The model under review builds one solid part; all positions refer to its coordinate system, in mm. A direction names the side the tool comes from. Coordinates: 2 decimals unless noted, no trailing zeros. Order: outer loops, then holes, each group sorted by start corner. A loop starts at its lowest first (then second) coordinate and runs counter-clockwise, first axis right, second up. Notation, with made-up numbers: M 23,46.25 L 73,46.25 A18 cw 73,57.25 Z; hole C -35,-26 d11. An arc over 180 degrees is marked long. Answer in a Markdown table with one row per item.
from build123d import *

# Parameters (mm, degrees)
ESQUISSE1_W             = 266.7
ESQUISSE1_H             = 38.1
BOSS_EXTRU_1_DEPTH      = 12.7
ESQUISSE2_W             = 12.7
ESQUISSE2_H             = 38.1
BOSS_EXTRU_2_DEPTH      = 279.4
ESQUISSE3_R             = 3.175
ENL_V_MAT_EXTRU_1_DEPTH = 311.176538442
ESQUISSE4_R             = 3.175
ENL_V_MAT_EXTRU_2_DEPTH = 311.176538442
BOSS_EXTRU_3_REACH      = 389.558
ESQUISSE5_W             = 38.1
ESQUISSE5_H             = 12.7
BOSS_EXTRU_4_REACH      = 389.558
ESQUISSE6_W             = 38.1
ESQUISSE6_H             = 12.7
ESQUISSE9_R             = 3.175
ENL_V_MAT_EXTRU_3_DEPTH = 396.997730423
ESQUISSE10_R            = 2
ENL_V_MAT_EXTRU_4_DEPTH = 396.997730423
ESQUISSE12_R            = 4.7625
ENL_V_MAT_EXTRU_5_DEPTH = 4.7625
ESQUISSE13_R            = 4.7625
ENL_V_MAT_EXTRU_6_DEPTH = 4.7625
ENL_V_START             = -76.2
ESQUISSE17_R            = 3.175
ENL_V_MAT_EXTRU_7_DEPTH = 76.2
ESQUISSE18_R            = 2
ENL_V_MAT_EXTRU_8_DEPTH = 25.4
ESQUISSE20_R            = 3.96875
ENL_V_MAT_EXTRU_9_DEPTH = 4.7625


with BuildPart() as part:
    # Esquisse1 → Boss.-Extru.1 (new body)
    with BuildSketch(Plane(origin=(0, 0, 0), x_dir=(1, 0, 0), z_dir=(0, 1, 0))):
        Rectangle(ESQUISSE1_W, ESQUISSE1_H)
    extrude(amount=BOSS_EXTRU_1_DEPTH)

    # Esquisse2 → Boss.-Extru.2 (add)
    with BuildSketch(Plane(origin=(0, 12.7, 0), x_dir=(1, 0, 0), z_dir=(0, 1, 0))):
        with Locations((-127, 0)):
            Rectangle(ESQUISSE2_W, ESQUISSE2_H)
        with Locations((127, 0)):
            Rectangle(ESQUISSE2_W, ESQUISSE2_H)
    extrude(amount=BOSS_EXTRU_2_DEPTH)

    # Esquisse3 → Enlèv. mat.-Extru.1 (cut, through all)
    with BuildSketch(Plane(origin=(0, 12.7, 0), x_dir=(1, 0, 0), z_dir=(0, 1, 0))):
        with Locations(Location((-22.225, 6.35, 0), (0, 0, 270))):
            Circle(ESQUISSE3_R)
    extrude(amount=-ENL_V_MAT_EXTRU_1_DEPTH, mode=Mode.SUBTRACT)

    # Esquisse4 → Enlèv. mat.-Extru.2 (cut, through all)
    with BuildSketch(Plane(origin=(0, 12.7, 0), x_dir=(1, 0, 0), z_dir=(0, 1, 0))):
        with Locations(Location((22.225, 6.35, 0), (0, 0, 270))):
            Circle(ESQUISSE4_R)
    extrude(amount=-ENL_V_MAT_EXTRU_2_DEPTH, mode=Mode.SUBTRACT)

    # Esquisse5 → Boss.-Extru.3 (add, up to next)
    with BuildSketch(Plane(origin=(-120.65, 0, 0), x_dir=(0, 0, -1), z_dir=(1, 0, 0)), mode=Mode.PRIVATE) as boss_extru_3_sk1:
        with Locations((0, 55.5625)):
            Rectangle(ESQUISSE5_W, ESQUISSE5_H)
    boss_extru_3_tool1 = extrude(boss_extru_3_sk1.sketch, amount=BOSS_EXTRU_3_REACH, mode=Mode.PRIVATE) - part.part
    add(boss_extru_3_tool1.solids().sort_by_distance((-120.65, 55.5625, 0))[0])

    # Esquisse6 → Boss.-Extru.4 (add, up to next)
    with BuildSketch(Plane(origin=(-120.65, 0, 0), x_dir=(0, 0, -1), z_dir=(1, 0, 0)), mode=Mode.PRIVATE) as boss_extru_4_sk1:
        with Locations((0, 285.75)):
            Rectangle(ESQUISSE6_W, ESQUISSE6_H)
    boss_extru_4_tool1 = extrude(boss_extru_4_sk1.sketch, amount=BOSS_EXTRU_4_REACH, mode=Mode.PRIVATE) - part.part
    add(boss_extru_4_tool1.solids().sort_by_distance((-120.65, 285.75, 0))[0])

    # Esquisse9 → Enlèv. mat.-Extru.3 (cut, through all)
    with BuildSketch(Plane.ZY.offset(133.35)):
        with Locations((0, 254)):
            Circle(ESQUISSE9_R)
    extrude(amount=-ENL_V_MAT_EXTRU_3_DEPTH, mode=Mode.SUBTRACT)

    # Esquisse10 → Enlèv. mat.-Extru.4 (cut, through all)
    with BuildSketch(Plane.ZY.offset(133.35)):
        with Locations((8, 262)):
            Circle(ESQUISSE10_R)
        with Locations((-8, 262)):
            Circle(ESQUISSE10_R)
        with Locations((-8, 246)):
            Circle(ESQUISSE10_R)
        with Locations((8, 246)):
            Circle(ESQUISSE10_R)
    extrude(amount=-ENL_V_MAT_EXTRU_4_DEPTH, mode=Mode.SUBTRACT)

    # Esquisse12 → Enlèv. mat.-Extru.5 (cut)
    with BuildSketch(Plane.ZY.offset(133.35)):
        with Locations((8, 262)):
            Circle(ESQUISSE12_R)
        with Locations((-8, 262)):
            Circle(ESQUISSE12_R)
        with Locations((-8, 246)):
            Circle(ESQUISSE12_R)
        with Locations((8, 246)):
            Circle(ESQUISSE12_R)
    extrude(amount=-ENL_V_MAT_EXTRU_5_DEPTH, mode=Mode.SUBTRACT)

    # Esquisse13 → Enlèv. mat.-Extru.6 (cut)
    with BuildSketch(Plane(origin=(120.65, 0, 0), x_dir=(0, 0, -1), z_dir=(1, 0, 0))):
        with Locations(Location((8, 262, 0), (0, 0, 180))):
            Circle(ESQUISSE13_R)
        with Locations(Location((8, 246, 0), (0, 0, 180))):
            Circle(ESQUISSE13_R)
        with Locations(Location((-8, 246, 0), (0, 0, 180))):
            Circle(ESQUISSE13_R)
        with Locations(Location((-8, 262, 0), (0, 0, 180))):
            Circle(ESQUISSE13_R)
    extrude(amount=ENL_V_MAT_EXTRU_6_DEPTH, mode=Mode.SUBTRACT)

    # Esquisse17 → Enlèv. mat.-Extru.7 (cut)
    with BuildSketch(Plane.XZ.offset(ENL_V_START)):
        with Locations(Location((22.225, -6.35, 0), (0, 0, 90))):
            Circle(ESQUISSE17_R)
        with Locations(Location((-22.225, -6.35, 0), (0, 0, 90))):
            Circle(ESQUISSE17_R)
    extrude(amount=ENL_V_MAT_EXTRU_7_DEPTH, mode=Mode.SUBTRACT)

    # Esquisse18 → Enlèv. mat.-Extru.8 (cut)
    with BuildSketch(Plane(origin=(0, 61.9125, 0), x_dir=(1, 0, 0), z_dir=(0, 1, 0))):
        with Locations(Location((14.225, -1.65, 0), (0, 0, 270))):
            Circle(ESQUISSE18_R)
        with Locations(Location((14.225, 14.35, 0), (0, 0, 270))):
            Circle(ESQUISSE18_R)
        with Locations(Location((30.225, 14.35, 0), (0, 0, 270))):
            Circle(ESQUISSE18_R)
        with Locations(Location((30.225, -1.65, 0), (0, 0, 270))):
            Circle(ESQUISSE18_R)
        with Locations(Location((-14.225, -1.65, 0), (0, 0, 270))):
            Circle(ESQUISSE18_R)
        with Locations(Location((-30.225, -1.65, 0), (0, 0, 270))):
            Circle(ESQUISSE18_R)
        with Locations(Location((-30.225, 14.35, 0), (0, 0, 270))):
            Circle(ESQUISSE18_R)
        with Locations(Location((-14.225, 14.35, 0), (0, 0, 270))):
            Circle(ESQUISSE18_R)
    extrude(amount=-ENL_V_MAT_EXTRU_8_DEPTH, mode=Mode.SUBTRACT)

    # Esquisse20 → Enlèv. mat.-Extru.9 (cut)
    with BuildSketch(Plane.XZ.offset(-49.2125)):
        with Locations(Location((30.225, -14.35, 0), (0, 0, 270))):
            Circle(ESQUISSE20_R)
        with Locations(Location((14.225, -14.35, 0), (0, 0, 270))):
            Circle(ESQUISSE20_R)
        with Locations(Location((14.225, 1.65, 0), (0, 0, 270))):
            Circle(ESQUISSE20_R)
        with Locations(Location((30.225, 1.65, 0), (0, 0, 270))):
            Circle(ESQUISSE20_R)
        with Locations(Location((-14.225, -14.35, 0), (0, 0, 270))):
            Circle(ESQUISSE20_R)
        with Locations(Location((-30.225, -14.35, 0), (0, 0, 270))):
            Circle(ESQUISSE20_R)
        with Locations(Location((-30.225, 1.65, 0), (0, 0, 270))):
            Circle(ESQUISSE20_R)
        with Locations(Location((-14.225, 1.65, 0), (0, 0, 270))):
            Circle(ESQUISSE20_R)
    extrude(amount=-ENL_V_MAT_EXTRU_9_DEPTH, mode=Mode.SUBTRACT)


solid = part.part
(1) The part is to be moulded in two halves that separate along Z. For faces 4 (the flat face through (120.65, 31, 0)), 5 (the cylindrical face through (-10.29, 51.56, 2.17)), 6 (the flat face through (-1, 59, -19.05)), say which applies: +Z half, -Z half, draft (parallel to the pull), parting line (faces both ways), or undercut.
Report:
| item | result |
|---|---|
| face 4 | draft |
| face 5 | undercut |
| face 6 | -Z half |
(2) To check wall thickness, follow line 1 (X direction, y = 9.5, z = -6.35); line 2 (Y direction, x = 110, z = -2); line 3 (Y direction, x = 131.25, z = -8). State the ranges of each line that lie inside material, in increasing order. Write a range as [from, to].
Report:
| item | result |
|---|---|
| line 1 | [-133.35, -25.4], [-19.05, 19.05], [25.4, 133.35] |
| line 2 | [0, 12.7], [49.21, 61.91], [279.4, 292.1] |
| line 3 | [0, 244], [248, 260], [264, 292.1] |
(3) Insertion check: P1, Ø11.5, axis at x = 30.5, z = -5.5, coming from the -Y side; P2, Ø4.5, axis at y = 246, z = -8, coming from the -X side. Each pin has a flat end and moves straight along its axis. Give the tip position at first contact, or say it passes through.
Report:
| item | result |
|---|---|
| P1 | y = 0 |
| P2 | x = -128.59 |
(4) Take a section at A-A (y = 176.5). Write out the cut boundary in (x, z).
Report:
| item | result |
|---|---|
| outline | M -133.35,-19.05 L -120.65,-19.05 L -120.65,19.05 L -133.35,19.05 Z; M 120.65,-19.05 L 133.35,-19.05 L 133.35,19.05 L 120.65,19.05 Z |
(5) Machinability: for faces 1 (the flat face through (125.413, 248, -7)), 2 (the cylindrical face through (19.077, 55.651, -6.763)), 3 (the cylindrical face through (-131, 250.72, 7.38)), which of the approach directions +Z, -Z, +X, -X, +Y, -Y give a long, thin tool a straight path to every point of the face, cutting with its end or side? Answer none if there is none.
Report:
| item | result |
|---|---|
| face 1 | none |
| face 2 | -Y |
| face 3 | -X |
(6) Take a section at B-B (x = -53). Write out the cut boundary in (y, z), then the cut area to 3 significant figures.
Report:
| item | result |
|---|---|
| outline | M 0,-19.05 L 12.7,-19.05 L 12.7,19.05 L 0,19.05 Z; M 49.21,-19.05 L 61.91,-19.05 L 61.91,19.05 L 49.21,19.05 Z; M 279.4,-19.05 L 292.1,-19.05 L 292.1,19.05 L 279.4,19.05 Z |
| area | 1,450 mm^2 |
